```python
from build123d import *

# Parameters (mm, degrees)
F1_DEPTH = 76
F2_W     = 23
F2_H     = 10.6
F2_R     = 1.15
F3_DEPTH = 1.4
F4_R     = 1.5
F5_DEPTH = 1.4


with BuildPart() as f1:
    # F0 (on Right) → F1 (new body)
    with BuildSketch(Plane.YZ):
        Polygon((0, 12), (0, 0), (1.4, 0), (1.4, 10.6), (12, 10.6), (12, 12), align=None)
    extrude(amount=F1_DEPTH)

    # F2 (on face) → F3 (cut, through all)
    with BuildSketch(Plane.XZ):
        with Locations((38, 5.3)):
            Rectangle(F2_W, F2_H)
        with Locations((24.01, 4.6)):
            Circle(F2_R)
        with Locations((51.99, 4.6)):
            Circle(F2_R)
    extrude(amount=-F3_DEPTH, mode=Mode.SUBTRACT)

    # F4 (on face) → F5 (cut, through all)
    with BuildSketch(Plane.XY.offset(12)):
        with Locations((6, 6)):
            Circle(F4_R)
        with Locations((70, 6)):
            Circle(F4_R)
    extrude(amount=-F5_DEPTH, mode=Mode.SUBTRACT)


solid = f1.part
```
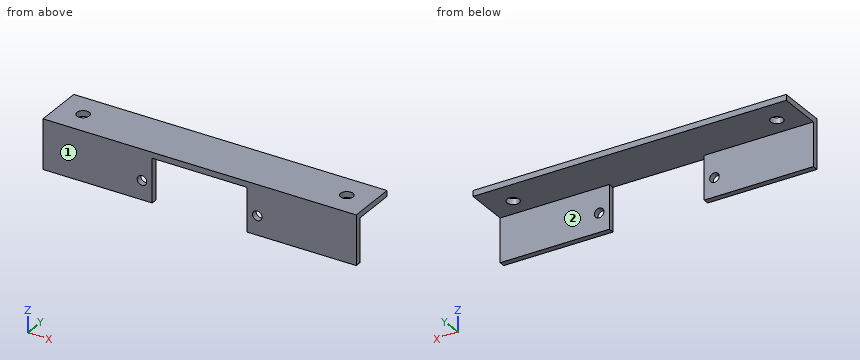
The listing builds one solid part. Answer for the finished solid, in the listing's coordinates (mm). Face numbers are marked on the shaded views. A direction names the side the tool comes from. Give positions to 0.01 mm unless a question says otherwise; leave off trailing zeros. Write each loop counter-clockwise with the first axis right and the second up, starting at its lowest first coordinate (ties: lowest second). Pieces come first, ordered by that corner, then holes. Notation, with made-up numbers: (33.5, 66) -> (49.5, 66) arc R32 ccw to (49.5, 105) -> close; hole circle Ø9 at (76.5, -5.5). An arc over 180 degrees is marked (long way). Write item = value, one per line. Start each with the question number.
1) The part is cut by section C-C, the plane z = 4.6. Determine the outline of the cut face in (x, y).
2) The part is cut by section A-A, the plane x = 51.99. Determine the outline of the cut face in (y, z), and give its area (3 significant figures).
3) The part is cut by section D-D, the plane x = 11.5. Determine the outline of the cut face in (y, z).
4) Each of these flat-tipped pins is pushed along its axis until it touches: pin 1 (2.5 mm diameter, centred on x = 24.01, z = 4.6, fed in from +Y); pin 2 (5 mm diameter, centred on x = 9.5, y = 5, fed in from -Z). Where does it stop, or does it pass through?
5) The part is cut by section B-B, the plane z = 8.5. Determine the outline of the cut face in (x, y), and give its area (3 significant figures).
6) Which of the six approach directions +Z, -Z, +X, -X, +Y, -Y give full straight-line access (tool end or side, diameter ignored) to the marked faces 1 and 2?
7) Straight lines are drawn through the part: line 1 along X through (y, z) = (6.75, 10.75); line 2 along Y through (x, z) = (70, 11.3); line 3 along Z through (x, y) = (63.5, 9.75). For each, find the intervals that lie inside material, in ascending order.
Solutions:
q1.outline = (0, 0) -> (22.86, 0) -> (22.86, 1.4) -> (0, 1.4) -> close; (25.16, 0) -> (26.5, 0) -> (26.5, 1.4) -> (25.16, 1.4) -> close; (49.5, 0) -> (50.84, 0) -> (50.84, 1.4) -> (49.5, 1.4) -> close; (53.14, 0) -> (76, 0) -> (76, 1.4) -> (53.14, 1.4) -> close
q2.outline = (0, 0) -> (1.4, 0) -> (1.4, 3.45) -> (0, 3.45) -> close; (0, 5.75) -> (1.4, 5.75) -> (1.4, 10.6) -> (12, 10.6) -> (12, 12) -> (0, 12) -> close
q2.area = 28.4 mm²
q3.outline = (0, 0) -> (1.4, 0) -> (1.4, 10.6) -> (12, 10.6) -> (12, 12) -> (0, 12) -> close
q4.pin_1 = 1.4
q4.pin_2 = 10.6
q5.outline = (0, 0) -> (26.5, 0) -> (26.5, 1.4) -> (0, 1.4) -> close; (49.5, 0) -> (76, 0) -> (76, 1.4) -> (49.5, 1.4) -> close
q5.area = 74.2 mm²
q6.face_1 = +Z, -Z, +X, -X, -Y
q6.face_2 = -Z, +X, -X, +Y
q7.line_1 = 0 to 4.7, 7.3 to 68.7, 71.3 to 76
q7.line_2 = 0 to 4.5, 7.5 to 12
q7.line_3 = 10.6 to 12
